Here's how the part is built. I have some questions about the finished solid (model axes, mm). Coordinates: 2 decimals unless noted, no trailing zeros. Loops run counter-clockwise (first coordinate to the right, second up) from the corner with the lowest first, then second, coordinate; pieces in that order, holes last. Notation, with made-up numbers: (58, -29.75) -> (107, -29.75) arc R18 cw to (107, -0.75) -> close; hole circle Ø2 at (-24.5, 11.25). An arc over 180 degrees is marked (long way). Answer as a JSON object with one key per item and string values. Group by question number.
Q1. I want a section at C-C on x = -21.25. Write out the boundary of the cut face in (y, z).
Q2. I need wall thicknesses on line 1 (Y direction, x = 21.25, z = 2); line 2 (Y direction, x = -22, z = 1.75); line 3 (X direction, y = 4, z = 1.1). Which ranges of each line are inside material? Lowest first, please.
Q3. Thinking about a two-plate mould opening in X: for faces 1 (the cylindrical face through (-49.584, 15.734, 2.535)), 2 (the cylindrical face through (41, 0, 2)), 3 (the cylindrical face through (49.234, 16.084, 2.535)), 4 (the flat face through (-0.8, 5.3, 0)), which applies, released by +X, released by -X, zero draft, split by the parting line, or undercut?
Q4. I want a section at D-D on y = -16. Write out the boundary of the cut face in (x, z).
Q5. I want a section at A-A on x = 0. Write out the boundary of the cut face in (y, z), then the cut area to 3 significant figures.
Q6. I want a section at B-B on z = 1.5. Count the separate pieces of the cut face and the enclosed holes in it, then the cut area to 3 significant figures.
Q7. I'm going to push flat-ended pins straight in: pin 1 (6 mm diameter, centred on x = 0, y = 0, fed in from -Z); pin 2 (5 mm diameter, centred on x = -16, y = 11, fed in from -Z); pin 3 (2 mm diameter, centred on y = 16, z = 2, fed in from -X). Where does each tip first touch, or does it pass through?
```python
from build123d import *

# Parameters (mm, degrees)
ESQUISSE1_W        = 112
ESQUISSE1_H        = 45
ESQUISSE1_R        = 1.75
ESQUISSE1_R_2      = 5
BOSS_EXTRU_1_DEPTH = 5
CONG_1_R           = 22.5


with BuildPart() as part:
    # Esquisse1 → Boss.-Extru.1 (new body)
    with BuildSketch(Plane.XY):
        Rectangle(ESQUISSE1_W, ESQUISSE1_H)
        with Locations((21.25, 0)):
            Circle(ESQUISSE1_R, mode=Mode.SUBTRACT)
        with Locations(Location((-21.25, 0, 0), (0, 0, 180))):
            Circle(ESQUISSE1_R, mode=Mode.SUBTRACT)
        with Locations((46, 0)):
            Circle(ESQUISSE1_R_2, mode=Mode.SUBTRACT)
        with Locations(Location((-46, 0, 0), (0, 0, 180))):
            Circle(ESQUISSE1_R_2, mode=Mode.SUBTRACT)
        Circle(ESQUISSE1_R_2, mode=Mode.SUBTRACT)
    extrude(amount=BOSS_EXTRU_1_DEPTH)

    # Congé1
    cong_1_edges = [part.edges().sort_by_distance(p)[0] for p in [
        (-56, -22.5, 2.5),
        (-56, 22.5, 2.5),
        (56, -22.5, 2.5),
        (56, 22.5, 2.5),
    ]]
    fillet(cong_1_edges, radius=CONG_1_R - 0.0001)  # a hair under: the kernel refuses the full size


solid = part.part
```
Result set:
{
 "1": {"outline": "(-22.5, 0) -> (-1.75, 0) -> (-1.75, 5) -> (-22.5, 5) -> close; (1.75, 0) -> (22.5, 0) -> (22.5, 5) -> (1.75, 5) -> close"},
 "2": {"line 1": "y = -22.5 to -1.75, 1.75 to 22.5", "line 2": "y = -22.5 to -1.58, 1.58 to 22.5", "line 3": "x = -55.64 to -49, -43 to -3, 3 to 43, 49 to 55.64"},
 "3": {"face 1": "released by -X", "face 2": "undercut", "face 3": "released by +X", "face 4": "zero draft"},
 "4": {"outline": "(-49.32, 0) -> (49.32, 0) -> (49.32, 5) -> (-49.32, 5) -> close"},
 "5": {"outline": "(-22.5, 0) -> (-5, 0) -> (-5, 5) -> (-22.5, 5) -> close; (5, 0) -> (22.5, 0) -> (22.5, 5) -> (5, 5) -> close", "area": "175 mm²"},
 "6": {"separate pieces": "1", "enclosed holes": "5", "area": "4,350 mm²"},
 "7": {"pin 1": "passes through", "pin 2": "stops at z = 0", "pin 3": "stops at x = -50.27"}
}
